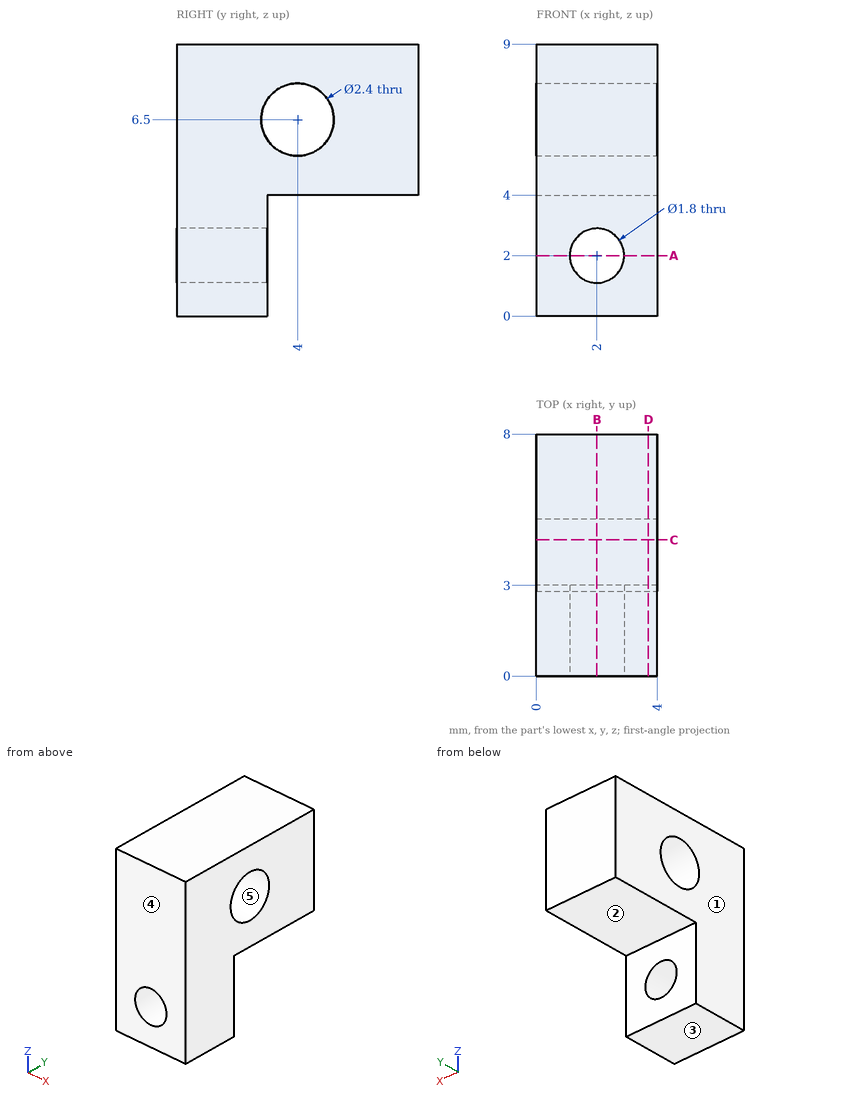
Job drawing, mm, ordinate dimensions from the low corner. One solid piece. A direction names the side the tool comes from. Coordinates: 2 decimals unless noted, no trailing zeros. Write each loop counter-clockwise with the first axis right and the second up, starting at its lowest first coordinate (ties: lowest second). Pieces come first, ordered by that corner, then holes.
Item 1: Slice it at D-D (x = 3.7). Write the cut outline in (y, z), and give its area (3 significant figures).
Item 2: Slice it at C-C (y = 4.5). Write the cut outline in (x, z), and give its area (3 significant figures).
Item 3: Which spindle directions (+Z, -Z, +X, -X, +Y, -Y) get a long thin tool onto all of the face, cutting with end or side? Do the marked faces 1 and 2. Say none if no direction does.
Item 4: Pin check, flat tip, straight feed: pin 1 (2 mm diameter, centred on x = 1.5, y = 5, fed in from -Z). Stop position of the tip, or through.
Item 5: Slice it at B-B (x = 2). Write the cut outline in (y, z), and give its area (3 significant figures).
Item 6: Probe line 1 (Z direction, x = 2, y = 1); line 2 (X direction, y = 2.1, z = 2); line 3 (Z direction, x = 1.9, y = 4). List the from-to ranges inside material, lowest first.
Item 7: Mould opens along Y. For the marked faces 3, 4 and 5 say: released by +Y, released by -Y, zero draft, split by the parting line, or undercut.
Item 8: Slice it at A-A (z = 2). Write the cut outline in (x, y).
Results found:
1. outline: (0, 0) - (3, 0) - (3, 4) - (8, 4) - (8, 9) - (0, 9) - close; hole circle Ø2.4 at (4, 6.5)
1. area: 47.5 mm2
2. outline: (0, 4) - (4, 4) - (4, 5.41) - (0, 5.41) - close; (0, 7.59) - (4, 7.59) - (4, 9) - (0, 9) - close
2. area: 11.3 mm2
3. face 1: +Z, -Z, -X, +Y, -Y
3. face 2: -Z, +X, -X, +Y
4. pin 1: stops at z = 4
5. outline: (0, 0) - (3, 0) - (3, 1.1) - (0, 1.1) - close; (0, 2.9) - (3, 2.9) - (3, 4) - (8, 4) - (8, 9) - (0, 9) - close; hole circle Ø2.4 at (4, 6.5)
5. area: 42.1 mm2
6. line 1: z = 0 to 1.1, 2.9 to 9
6. line 2: x = 0 to 1.1, 2.9 to 4
6. line 3: z = 4 to 5.3, 7.7 to 9
7. face 3: zero draft
7. face 4: released by -Y
7. face 5: undercut
8. outline: (0, 0) - (1.1, 0) - (1.1, 3) - (0, 3) - close; (2.9, 0) - (4, 0) - (4, 3) - (2.9, 3) - close
